Verification items for this drawing (mm, ordinates from the low corner). Give positions to 0.01 mm unless a question says otherwise; leave off trailing zeros. Order: outer loops, then holes, each group sorted by start corner. A loop starts at its lowest first (then second) coordinate and runs counter-clockwise, first axis right, second up. Notation, with made-up numbers: M 48.25,-1 L 65.25,-1 A19 cw 65.25,10 Z; hole C -30,89 d8. An arc over 180 degrees is marked long. Answer as a JSON object with one key per item and string values.
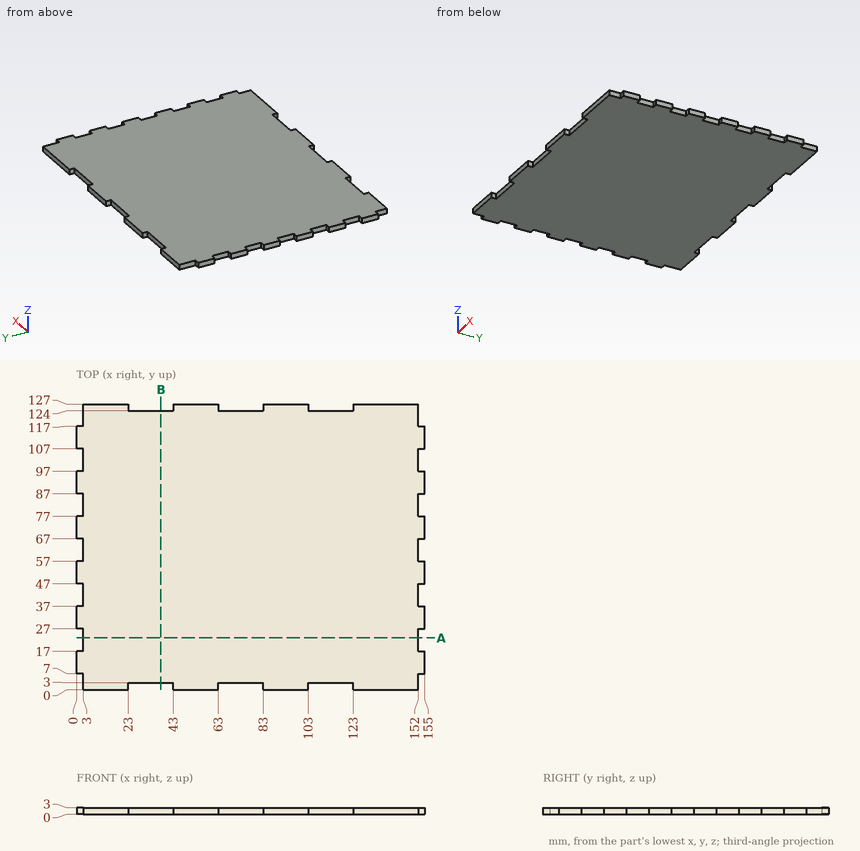
Q1. Gauge pin test, flat ends, axial feed: pin 1 Ø0.9 at (y, z) = (41.5, 1) entering from -X; pin 2 Ø1.5 at (x, z) = (1.5, 1.5) entering from -Y; pin 3 Ø1.5 at (y, z) = (42.5, 2) entering from +X. Record the tip position at first contact, or that the pin passes through.
Resolved:
{"pin 1": "stops at x = 3", "pin 2": "stops at y = 7", "pin 3": "stops at x = 152"}
Q2. Material ranges on L1, parallel to X at y = 38, z = 1.8; L2, parallel to Y at x = 117.5, z = 2.85, recorded low to high.
Resolved:
{"L1": "x = 3 to 152", "L2": "y = 3 to 124"}
Q3. Section check B-B on x = 37.5. Record the cut outline in (y, z).
Resolved:
{"outline": "M 3,0 L 124,0 L 124,3 L 3,3 Z"}
Q4. Section check A-A on y = 23. Record the cut outline in (x, z).
Resolved:
{"outline": "M 3,0 L 152,0 L 152,3 L 3,3 Z"}
